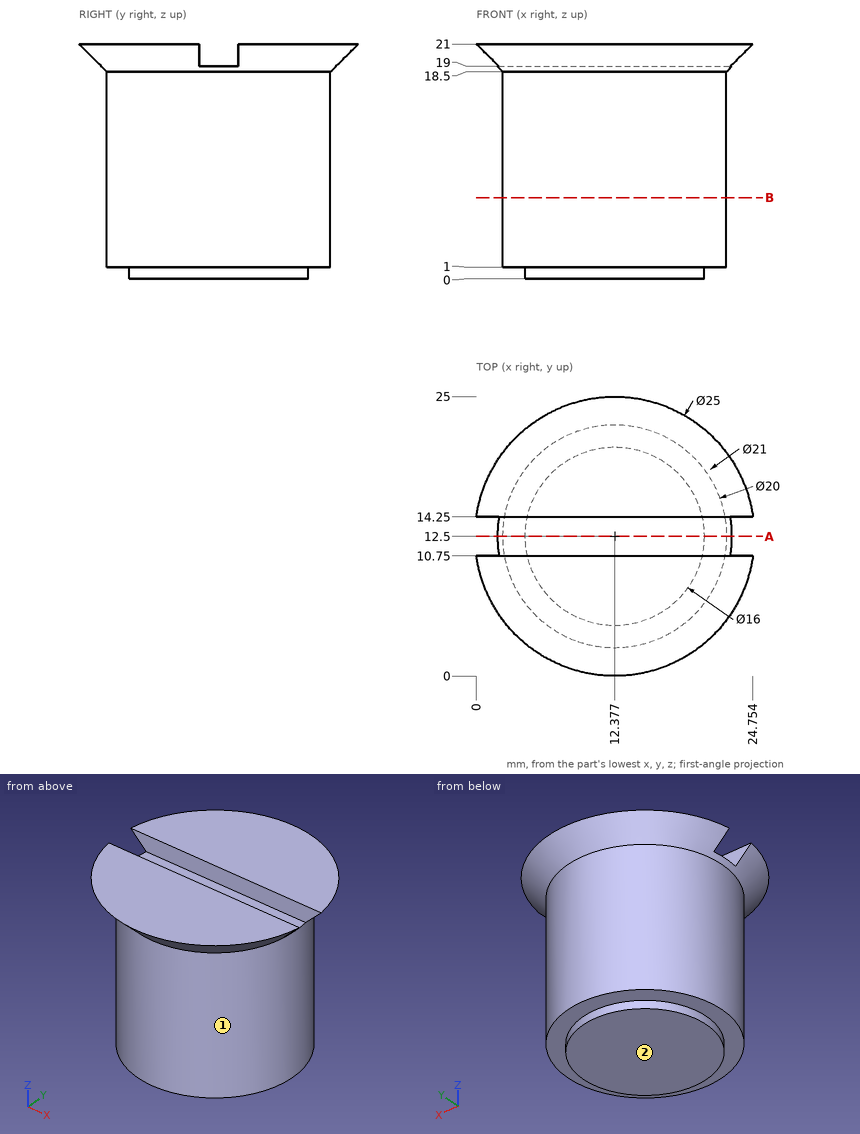
Geometry check sheet. Reference: drawing and pictorial views, mm from the part's lowest x, y, z. A direction names the side the tool comes from. Coordinates: 2 decimals unless noted, no trailing zeros. Order: outer loops, then holes, each group sorted by start corner. A loop starts at its lowest first (then second) coordinate and runs counter-clockwise, first axis right, second up.
Item 1: Scan lines: line 1 along Y through (x, z) = (13.25, 9.5); line 2 along Z through (x, y) = (11.25, 2.5); line 3 along Y through (x, z) = (5.75, 18.75). Record each from-to range of solid material in increasing order.
Item 2: Section check A-A (y = 12.5). Enter the section's corners in (x, z), plus the area to 3 significant figures.
Item 3: Section check B-B (z = 7.25). Enter the section's corners in (x, y).
Item 4: Tool access check on the marked faces 1 and 2. Record the directions out of +Z, -Z, +X, -X, +Y, -Y that give a thin tool (end or side, any length) a straight path to the whole face; none if there is none.
Item 5: Depth check by flat-ended pin: pin 1 (1 mm diameter, centred on x = 15.5, z = 7, fed in from +Y); pin 2 (5 mm diameter, centred on y = 18.5, z = 11.5, fed in from -X); pin 3 (2 mm diameter, centred on x = 6.5, z = 5, fed in from +Y). Enter the tip coordinate at first touch or a pass-through.
Check sheet entries:
1. line 1: y = 2.54 to 22.46
1. line 2: z = 18.56 to 21
1. line 3: y = 4.68 to 20.32
2. outline: (1.88, 19) - (2.38, 18.5) - (2.38, 1) - (4.38, 1) - (4.38, 0) - (20.38, 0) - (20.38, 1) - (22.38, 1) - (22.38, 18.5) - (22.88, 19) - close
2. area: 376 mm2
3. outline: circle Ø20 at (12.38, 12.5)
4. face 1: -Z
4. face 2: -Z, +X, -X, +Y, -Y
5. pin 1: stops at y = 22.15
5. pin 2: stops at x = 3.01
5. pin 3: stops at y = 21.23
